Read the model definition and answer for the solid it produces. Units are mm, in the model's axes. Round coordinates to 2 decimals unless told otherwise and drop trailing zeros. Order: outer loops, then holes, each group sorted by start corner. A loop starts at its lowest first (then second) coordinate and runs counter-clockwise, first axis right, second up. Notation, with made-up numbers: M 11.5,-29 L 39.5,-29 A14 ccw 39.5,-7 Z; hole C -21,-6.75 d3. An arc over 180 degrees is marked long. Answer as CSV lines item,"result".
```python
from build123d import *

# Parameters (mm, degrees)
BASPROSKE_W         = 12
BASPROSKE_H         = 12
TOOTHCUT_DEPTH      = 21.784609691
TEETHCUTS_COUNT     = 10
TEETHCUTS_ANGLE     = 324
BORSKE_R            = 2
BORE_DEPTH          = 50.0000508
CUT_EXTRUDE_1_DEPTH = 5


with BuildPart() as part:
    # BasProSke → Base-Revolve (revolve)
    with BuildSketch(Plane(origin=(0, 0, 0), x_dir=(1, 0, 0), z_dir=(0, 1, 0)), mode=Mode.PRIVATE) as base_revolve_sk:
        with Locations((6, 6)):
            Rectangle(BASPROSKE_W, BASPROSKE_H)
    revolve(base_revolve_sk.sketch.rotate(Axis((-10, 0, 0), (1, 0, 0)), 180), axis=Axis((-10, 0, 0), (1, 0, 0)))

    # TooCutSke → ToothCut (cut, through all)
    with BuildSketch(Plane(origin=(0, 0, 0), x_dir=(0, 0, -1), z_dir=(1, 0, 0))):
        with BuildLine():
            ThreePointArc((1.173662691, 7.406586048), (0, 7.499), (-1.173662691, 7.406586048))
            ThreePointArc((-1.173662691, 7.406586048), (-1.668191438, 9.834565786), (-3.497907776, 11.50542856))
            ThreePointArc((-3.497907776, 11.50542856), (0, 12.0254), (3.497907776, 11.50542856))
            ThreePointArc((3.497907776, 11.50542856), (1.668191438, 9.834565786), (1.173662691, 7.406586048))
        make_face()
    toothcut = extrude(amount=TOOTHCUT_DEPTH, mode=Mode.SUBTRACT)

    # TeethCuts: ToothCut ×10 about axis
    teethcuts_axis = Axis((-10, 0, 0), (1, 0, 0))
    for i in range(1, TEETHCUTS_COUNT):
        add(toothcut.rotate(teethcuts_axis, i * TEETHCUTS_ANGLE / (TEETHCUTS_COUNT - 1)), mode=Mode.SUBTRACT)

    # BorSke → Bore (cut, symmetric)
    with BuildSketch(Plane(origin=(0, 0, 0), x_dir=(0, 0, -1), z_dir=(1, 0, 0))):
        with Locations(Location((0, 0, 0), (0, 0, 180))):
            Circle(BORSKE_R)
    extrude(amount=BORE_DEPTH, both=True, mode=Mode.SUBTRACT)

    # Эскиз1 → Вырез-Вытянуть1 (cut)
    with BuildSketch(Plane.ZY):
        Polygon((7.505553499, 0), (3.75277675, 6.5), (-3.75277675, 6.5), (-7.505553499, 0), (-3.75277675, -6.5), (3.75277675, -6.5), align=None)
    extrude(amount=-CUT_EXTRUDE_1_DEPTH, mode=Mode.SUBTRACT)


solid = part.part
```
Item 1: A cutting plane is placed at D-D, the plane y = -4.75. Determine the outline of the cut face in (x, z), and give its area (3 significant figures).
Ans:
outline,"M 0,-8.95 L 12,-8.95 L 12,8.95 L 0,8.95 L 0,4.76 L 5,4.76 L 5,-4.76 L 0,-4.76 Z"
area,"167 mm2"
Item 2: A cutting plane is placed at C-C, the plane z = -8.75. Determine the outline of the cut face in (x, y).
Ans:
outline,"M 0,-7.33 L 12,-7.33 L 12,-4.53 L 0,-4.53 Z; M 0,-1.52 L 12,-1.52 L 12,1.52 L 0,1.52 Z; M 0,4.53 L 12,4.53 L 12,7.33 L 0,7.33 Z"
Item 3: Determine the mould class of faces 1 (the face through (0, -7, 0)), 2 (the face through (2, 6.5, 0)) for opening direction Z: +Z half, -Z half, draft (parallel to the pull), parting line (faces both ways), or undercut.
Ans:
face 1,"draft"
face 2,"undercut"
Item 4: A cutting plane is placed at B-B, the plane y = 8.75. Determine the outline of the cut face in (x, z).
Ans:
outline,"M 0,-4.41 L 12,-4.41 L 12,-1.25 L 0,-1.25 Z; M 0,1.25 L 12,1.25 L 12,4.41 L 0,4.41 Z"
Item 5: Flat-ended cylindrical pins translate along their axes: pin 1 (1.5 mm diameter, centred on x = 2, z = 1.5, fed in from +Y); pin 2 (1.5 mm diameter, centred on y = -8.5, z = 5, fed in from +X); pin 3 (3 mm diameter, centred on x = 8, y = 7.5, fed in from -Z); pin 4 (4 mm diameter, centred on x = 4, z = 5, fed in from -Y). Find the tip coordinate at first contact, or state that the pin passes through.
Ans:
pin 1,"y = 10.62"
pin 2,"x = 12"
pin 3,"z = -9.86"
pin 4,"y = -11.49"
Item 6: A cutting plane is placed at A-A, the plane z = 0. Determine the outline of the cut face in (x, y), and give its area (3 significant figures).
Ans:
outline,"M 0,-7.5 L 12,-7.5 L 12,-2 L 5,-2 L 5,-6.5 L 0,-6.5 Z; M 0,6.5 L 5,6.5 L 5,2 L 12,2 L 12,7.5 L 0,7.5 Z"
area,"87.0 mm2"
Item 7: Find the intervals of material crossed by probe 1 along Y at (x, z) = (10.25, 0); probe 2 along Y at (x, z) = (7.75, 9); probe 3 along Z at (x, y) = (3.5, -7), in increasing order. Write a range as [from, to].
Ans:
probe 1,"[-7.5, -2], [2, 7.5]"
probe 2,"[-7.33, -4.81], [-1.53, 1.53], [4.81, 7.33]"
probe 3,"[-9.75, -7.18], [-3.67, 3.67], [7.18, 9.75]"
